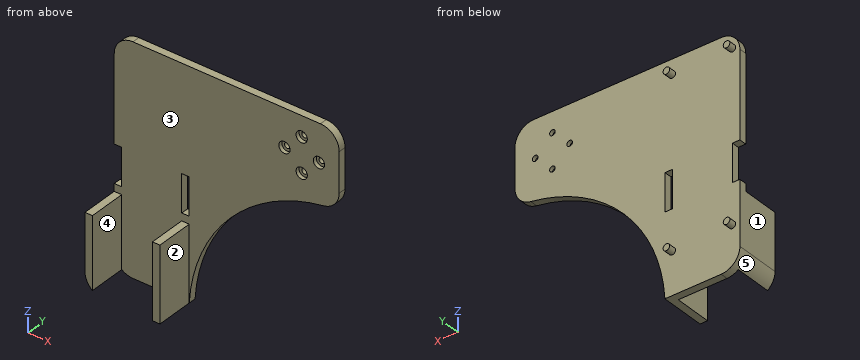
from build123d import *

# Parameters (mm, degrees)
SKETCH1_R           = 0.9525
BOSS_EXTRUDE1_DEPTH = 2.54
SKETCH2_W           = 2.54
SKETCH2_H           = 25.4
BOSS_EXTRUDE2_DEPTH = 12.7
FILLET2_R           = 6.35
FILLET3_R           = 6.35
FILLET4_R           = 6.35
FILLET5_R           = 6.35
SKETCH3_R           = 1.905
CUT_EXTRUDE1_DEPTH  = 1.27
SKETCH4_W           = 2.54
SKETCH4_H           = 12.7
CUT_EXTRUDE2_DEPTH  = 109.508847566
SKETCH5_R           = 1.1176
BOSS_EXTRUDE3_DEPTH = 2.54


with BuildPart() as part:
    # Sketch1 → Boss-Extrude1 (new body)
    with BuildSketch(Plane(origin=(0, 0, 0), x_dir=(1, 0, 0), z_dir=(0, 1, 0))):
        with BuildLine():
            Line((0, 0), (0, 76.2))
            Line((0, 76.2), (25.4, 76.2))
            ThreePointArc((25.4, 76.2), (41.142937212, 41.142937212), (76.2, 25.4))
            Line((76.2, 25.4), (76.2, 0))
            Line((76.2, 0), (0, 0))
        make_face()
        with Locations(Location((63.5, 6.858, 0), (0, 0, 270))):
            Circle(SKETCH1_R, mode=Mode.SUBTRACT)
        with Locations(Location((57.658, 12.7, 0), (0, 0, 270))):
            Circle(SKETCH1_R, mode=Mode.SUBTRACT)
        with Locations(Location((63.5, 18.542, 0), (0, 0, 270))):
            Circle(SKETCH1_R, mode=Mode.SUBTRACT)
        with Locations(Location((69.342, 12.7, 0), (0, 0, 270))):
            Circle(SKETCH1_R, mode=Mode.SUBTRACT)
    extrude(amount=BOSS_EXTRUDE1_DEPTH)

    # Sketch2 → Boss-Extrude2 (add)
    with BuildSketch(Plane.XZ):
        with Locations((1.27, -63.5)):
            Rectangle(SKETCH2_W, SKETCH2_H)
        with Locations((24.13, -63.5)):
            Rectangle(SKETCH2_W, SKETCH2_H)
    extrude(amount=BOSS_EXTRUDE2_DEPTH)

    # Fillet2
    fillet2_edges = [part.edges().sort_by_distance(p)[0] for p in [
        (0, -5.08, -76.2),
    ]]
    fillet(fillet2_edges, radius=FILLET2_R)

    # Fillet3
    fillet3_edges = [part.edges().sort_by_distance(p)[0] for p in [
        (0, 1.27, 0),
    ]]
    fillet(fillet3_edges, radius=FILLET3_R)

    # Fillet4
    fillet4_edges = [part.edges().sort_by_distance(p)[0] for p in [
        (76.2, 1.27, 0),
    ]]
    fillet(fillet4_edges, radius=FILLET4_R)

    # Fillet5
    fillet5_edges = [part.edges().sort_by_distance(p)[0] for p in [
        (76.2, 1.27, -25.4),
    ]]
    fillet(fillet5_edges, radius=FILLET5_R)

    # Sketch3 → Cut-Extrude1 (cut)
    with BuildSketch(Plane.XZ):
        with Locations(Location((63.5, -6.858, 0), (0, 0, 270))):
            Circle(SKETCH3_R)
        with Locations(Location((69.342, -12.7, 0), (0, 0, 270))):
            Circle(SKETCH3_R)
        with Locations(Location((57.658, -12.7, 0), (0, 0, 270))):
            Circle(SKETCH3_R)
        with Locations(Location((63.5, -18.542, 0), (0, 0, 270))):
            Circle(SKETCH3_R)
    extrude(amount=-CUT_EXTRUDE1_DEPTH, mode=Mode.SUBTRACT)

    # Sketch4 → Cut-Extrude2 (cut, through all)
    with BuildSketch(Plane.XZ):
        with Locations((24.13, -41.91)):
            Rectangle(SKETCH4_W, SKETCH4_H)
        with Locations((1.27, -41.91)):
            Rectangle(SKETCH4_W, SKETCH4_H)
    extrude(amount=-CUT_EXTRUDE2_DEPTH, mode=Mode.SUBTRACT)

    # Sketch5 → Boss-Extrude3 (add)
    with BuildSketch(Plane(origin=(0, 2.54, 0), x_dir=(1, 0, 0), z_dir=(0, 1, 0))):
        with Locations(Location((2.54, 5.08, 0), (0, 0, 270))):
            Circle(SKETCH5_R)
        with Locations(Location((2.54, 61.96076, 0), (0, 0, 270))):
            Circle(SKETCH5_R)
        with Locations(Location((22.92096, 61.96076, 0), (0, 0, 270))):
            Circle(SKETCH5_R)
        with Locations(Location((22.92096, 5.08, 0), (0, 0, 270))):
            Circle(SKETCH5_R)
    extrude(amount=BOSS_EXTRUDE3_DEPTH)


solid = part.part
Geometry: final body of the model. Coordinates: model frame, mm. Face numbers are marked on the shaded views. A direction names the side the tool comes from. Coordinates: 2 decimals unless noted, no trailing zeros. Order: outer loops, then holes, each group sorted by start corner. A loop starts at its lowest first (then second) coordinate and runs counter-clockwise, first axis right, second up.
(1) First-contact query: pin 1 (3 mm diameter, centred on y = 0.5, z = -42.5, fed in from -X); pin 2 (1.3 mm diameter, centred on y = 1, z = -40, fed in from +X); pin 3 (3 mm diameter, centred on x = 57.658, z = -12.7, fed in from +Y). Flat tips, straight axial feed; report the tip coordinate or a pass-through.
(2) Draft query along X for the marked faces 1, 2 and 3. Return one class per face: pulls with the +X half, pulls with the -X half, needs draft (parallel to the pull), parting line crosses it, or undercut.
(3) Section query B-B (y = -5). Return the cut outline in (x, z).
(4) Section query A-A (z = -12.7). Return the cut outline in (x, y).
(5) Access query for the marked faces 4 and 5. Directions: +Z, -Z, +X, -X, +Y, -Y. A direction counts if a zero-diameter tool reaches every point of the face in a straight line with its end or side. Return the directions, or none.
(6) Material intervals for probe 1 along X at (y, z) = (2.2, -12.7); probe 2 along X at (y, z) = (-3, -58); probe 3 along Z at (x, y) = (23.5, 1.5), sorted ascending.
(7) Section query D-D (z = -37). Return the cut outline in (x, y), plus the area to 3 significant figures.
(8) Section query C-C (x = 63.5). Return the cut outline in (y, z), plus the area to 3 significant figures.
Solution:
1. pin 1: stops at x = 2.54
1. pin 2: stops at x = 43.02
1. pin 3: stops at y = 2.54
2. face 1: pulls with the -X half
2. face 2: pulls with the +X half
2. face 3: undercut
3. outline: (0, -69.85) arc R6.35 ccw to (2.54, -74.93) - (2.54, -50.8) - (0, -50.8) - close; (22.86, -76.2) - (25.4, -76.2) - (25.4, -50.8) - (22.86, -50.8) - close
4. outline: (0, 0) - (55.75, 0) - (55.75, 1.27) - (56.71, 1.27) - (56.71, 2.54) - (0, 2.54) - close; (58.61, 1.27) - (59.56, 1.27) - (59.56, 0) - (67.44, 0) - (67.44, 1.27) - (68.39, 1.27) - (68.39, 2.54) - (58.61, 2.54) - close; (70.29, 1.27) - (71.25, 1.27) - (71.25, 0) - (76.2, 0) - (76.2, 2.54) - (70.29, 2.54) - close
5. face 4: +Z, -Z, -Y
5. face 5: -Z, -X, +Y, -Y
6. probe 1: x = 0 to 56.71, 58.61 to 68.39, 70.29 to 76.2
6. probe 2: x = 0 to 2.54, 22.86 to 25.4
6. probe 3: z = -76.2 to -48.26, -35.56 to 0
7. outline: (2.54, 0) - (22.86, 0) - (22.86, 2.54) - (2.54, 2.54) - close; (25.4, 0) - (45.79, 0) - (45.79, 2.54) - (25.4, 2.54) - close
7. area: 103 mm2
8. outline: (0, -27.69) - (2.54, -27.69) - (2.54, -19.49) - (1.27, -19.49) - (1.27, -20.45) - (0, -20.45) - close; (0, -16.64) - (1.27, -16.64) - (1.27, -17.59) - (2.54, -17.59) - (2.54, -7.81) - (1.27, -7.81) - (1.27, -8.76) - (0, -8.76) - close; (0, -4.95) - (1.27, -4.95) - (1.27, -5.91) - (2.54, -5.91) - (2.54, 0) - (0, 0) - close
8. area: 55.8 mm2
